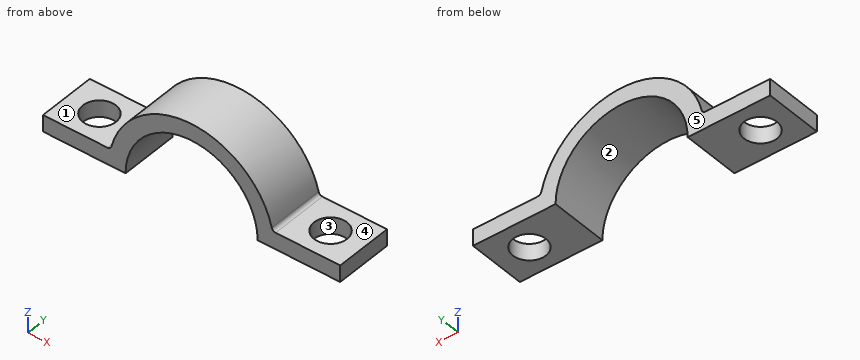
from build123d import *

# Parameters (mm, degrees)
BOSS_EXTRUDE1_DEPTH = 5.5626
SKETCH2_R           = 3.175
CUT_EXTRUDE1_DEPTH  = 32.761031843


with BuildPart() as part:
    # Sketch1 → Boss-Extrude1 (new, symmetric)
    with BuildSketch(Plane(origin=(0, 0, 0), x_dir=(1, 0, 0), z_dir=(0, 1, 0))):
        with BuildLine():
            Line((-12.7, 0), (-28.575, 0))
            Line((-28.575, 0), (-28.575, -3.175))
            Line((-28.575, -3.175), (-16.164461018, -3.175))
            ThreePointArc((-16.164461018, -3.175), (-15.693695846, -3.337813758), (-15.424104025, -3.756679389))
            ThreePointArc((-15.424104025, -3.756679389), (0, -15.875), (15.424104025, -3.756679389))
            ThreePointArc((15.424104025, -3.756679389), (15.693695846, -3.337813758), (16.164461018, -3.175))
            Line((16.164461018, -3.175), (28.575, -3.175))
            Line((28.575, -3.175), (28.575, 0))
            Line((28.575, 0), (12.7, 0))
            ThreePointArc((12.7, 0), (0, -12.7), (-12.7, 0))
        make_face()
    extrude(amount=BOSS_EXTRUDE1_DEPTH, both=True)

    # Sketch2 → Cut-Extrude1 (cut, through all)
    with BuildSketch(Plane.XY.offset(3.175)):
        with Locations((-22.225, 0)):
            Circle(SKETCH2_R)
        with Locations((22.225, 0)):
            Circle(SKETCH2_R)
    extrude(amount=-CUT_EXTRUDE1_DEPTH, mode=Mode.SUBTRACT)


solid = part.part
Can you work these out from the model? Positions are in its coordinate system, mm. Face numbers are marked on the shaded views. A direction names the side the tool comes from. Give positions to 0.01 mm unless a question says otherwise; leave off trailing zeros. Loops run counter-clockwise (first coordinate to the right, second up) from the corner with the lowest first, then second, coordinate; pieces in that order, holes last. Notation, with made-up numbers: (-39, 33) - (-10, 33) arc R16 ccw to (-10, 43) - close; hole circle Ø11 at (23.25, -33). An arc over 180 degrees is marked (long way). One line per item, written item: value.
(1) I'm going to push flat-ended pins straight in: pin 1 (6 mm diameter, centred on y = -3.5, z = 10, fed in from +X); pin 2 (1 mm diameter, centred on y = -1, z = 13, fed in from -X); pin 3 (3.5 mm diameter, centred on x = 21.5, y = 0, fed in from +Z). Where does each tip first touch, or does it pass through?
Verdict:
pin 1: x = 14.25
pin 2: x = -9.79
pin 3: through
(2) If we section it at D-D, the plane x = 0: List the corners of the cut face in (y, z) for me (3 decimals).
Verdict:
outline: (-5.563, 12.7) - (5.563, 12.7) - (5.563, 15.875) - (-5.563, 15.875) - close
(3) I need wall thicknesses on line 1 along X through (y, z) = (3.5, 6.25); line 2 along X through (y, z) = (-0.75, 3) (3 decimals); line 3 along Y through (x, z) = (20, 1.25). Which ranges of each line are inside material? Lowest first, please.
Verdict:
line 1: -14.59 to -11.06, 11.06 to 14.59
line 2: -28.575 to -25.31, -19.14 to -12.341, 12.341 to 19.14, 25.31 to 28.575
line 3: -5.56 to -2.26, 2.26 to 5.56
(4) If we mould it in two halves opening along Y, with no side actions, what happens to the marked faces 3, 4 and 5? For each: released by +Y, released by -Y, zero draft, split by the parting line, or undercut.
Verdict:
face 3: undercut
face 4: zero draft
face 5: released by +Y
(5) If we section it at B-B, the plane z = 6: List the corners of the cut face in (x, y) for me.
Verdict:
outline: (-14.7, -5.56) - (-11.19, -5.56) - (-11.19, 5.56) - (-14.7, 5.56) - close; (11.19, -5.56) - (14.7, -5.56) - (14.7, 5.56) - (11.19, 5.56) - close
(6) On a 3-axis mill with a long thin cutter (end or side, diameter ignored), from which of +Z, -Z, +X, -X, +Y, -Y can I reach the whole of each face in a straight line? I mean the marked faces 1 and 2. Say none if no direction works.
Verdict:
face 1: +Z, -X, +Y, -Y
face 2: -Z, +Y, -Y
(7) If we section it at C-C, the plane y = 4.75: List the corners of the cut face in (x, z) for me (3 decimals).
Verdict:
outline: (-28.575, 0) - (-12.7, 0) arc R12.7 cw to (12.7, 0) - (28.575, 0) - (28.575, 3.175) - (16.164, 3.175) arc R0.762 cw to (15.424, 3.757) arc R15.875 ccw to (-15.424, 3.757) arc R0.762 cw to (-16.164, 3.175) - (-28.575, 3.175) - close
(8) If we section it at A-A, the plane y = 0: List the corners of the cut face in (x, z) for me (3 decimals).
Verdict:
outline: (-28.575, 0) - (-25.4, 0) - (-25.4, 3.175) - (-28.575, 3.175) - close; (-19.05, 0) - (-12.7, 0) arc R12.7 cw to (12.7, 0) - (19.05, 0) - (19.05, 3.175) - (16.164, 3.175) arc R0.762 cw to (15.424, 3.757) arc R15.875 ccw to (-15.424, 3.757) arc R0.762 cw to (-16.164, 3.175) - (-19.05, 3.175) - close; (25.4, 0) - (28.575, 0) - (28.575, 3.175) - (25.4, 3.175) - close
